from build123d import *

# Parameters (mm, degrees)
F1_R      = 2.5
F3_SIZE   = 2
F2_FACE_R = 0.5


with BuildPart() as f2:
    # F2: sweep along a path in F0
    with BuildLine(Plane.XZ) as f2_path:
        Line((0, 40.1438838244), (20, 40.1438838244))
        Line((20, 40.1438838244), (115.2627944163, -14.8561161756))
    # F1 (on Right) → F2 (sweep)
    with BuildSketch(Plane.YZ):
        with Locations((0, 40.1438838244)):
            Circle(F1_R)
    sweep(path=f2_path.line, transition=Transition.RIGHT)

    # F3
    f3_edges = [f2.edges().sort_by_distance(p)[0] for p in [
        (0, -2.5, 40.143884),
    ]]
    chamfer(f3_edges, length=F3_SIZE)

    # F4: sweep along a path in F0
    with BuildLine(Plane.XZ) as f4_path:
        Line((0, 40.1438838244), (20, 40.1438838244))
        Line((20, 40.1438838244), (115.2627944163, -14.8561161756))
    # F2_face (on face) → F4 (sweep, cut)
    with BuildSketch(Plane(origin=(0, 0, 40.1438838244), x_dir=(0, -1, 0), z_dir=(-1, 0, 0))):
        Circle(F2_FACE_R)
    sweep(path=f4_path.line, transition=Transition.RIGHT, mode=Mode.SUBTRACT)


solid = f2.part
Here's how the part is built. I have some questions about the finished solid (model axes, mm). A direction names the side the tool comes from. Give positions to 0.01 mm unless a question says otherwise; leave off trailing zeros. Answer as a JSON object with one key per item and string values. Group by question number.
1) I'm going to push flat-ended pins straight in: pin 1 Ø1.5 at (x, y) = (74, -1) entering from +Z; pin 2 Ø1 at (x, y) = (74.5, 1.5) entering from +Z. Where does each tip first touch, or does it pass through?
2) Please list where these lines run through material, in increasing order: L1, parallel to Z at x = 9.5, y = 0; L2, parallel to Z at x = 24, y = -0.4; L3, parallel to Y at x = 11, z = 38. Write a range as [from, to].
3) We'd pull the mould along Z, two halves only. Please class faces 3 (the cylindrical face through (68.49, 0.11, 12.71)), 4 (the flat face through (115.52, 0.52, -14.41)), 5 (the conical face through (0.32, 0.78, 40.39)): pulls with the +Z half, pulls with the -Z half, needs draft (parallel to the pull), parting line crosses it, or undercut.
4) On a 3-axis mill with a long thin cutter (end or side, diameter ignored), from which of +Z, -Z, +X, -X, +Y, -Y can I reach the whole of each face in a straight line? I mean faces 1 (the cylindrical face through (69.25, -0.33, 14.57)), 2 (the cylindrical face through (11.47, -0.33, 42.62)). Say none if no direction works.
Results found:
{
 "1": {"pin 1": "z = 12.14", "pin 2": "z = 11.45"},
 "2": {"L1": "[37.64, 39.64], [40.64, 42.64]", "L2": "[34.98, 37.49], [38.18, 40.68]", "L3": "[-1.29, 1.29]"},
 "3": {"face 3": "undercut", "face 4": "pulls with the -Z half", "face 5": "parting line crosses it"},
 "4": {"face 1": "none", "face 2": "-X"}
}
